Input: dimensioned drawing with shaded views. Units: mm. Origin: part minimum x, y, z. A direction names the side the tool comes from. Give positions to 0.01 mm unless a question says otherwise; leave off trailing zeros. Write each loop counter-clockwise with the first axis right and the second up, starting at its lowest first coordinate (ties: lowest second). Pieces come first, ordered by that corner, then holes. Notation, with made-up numbers: M -32.75,-15.75 L -12.75,-15.75 A23 ccw -12.75,16.25 Z; hole C -6,55.5 d7. An arc over 180 degrees is marked long. Use CSV: the item, a comma, the result in double quotes. Start each with the question number.
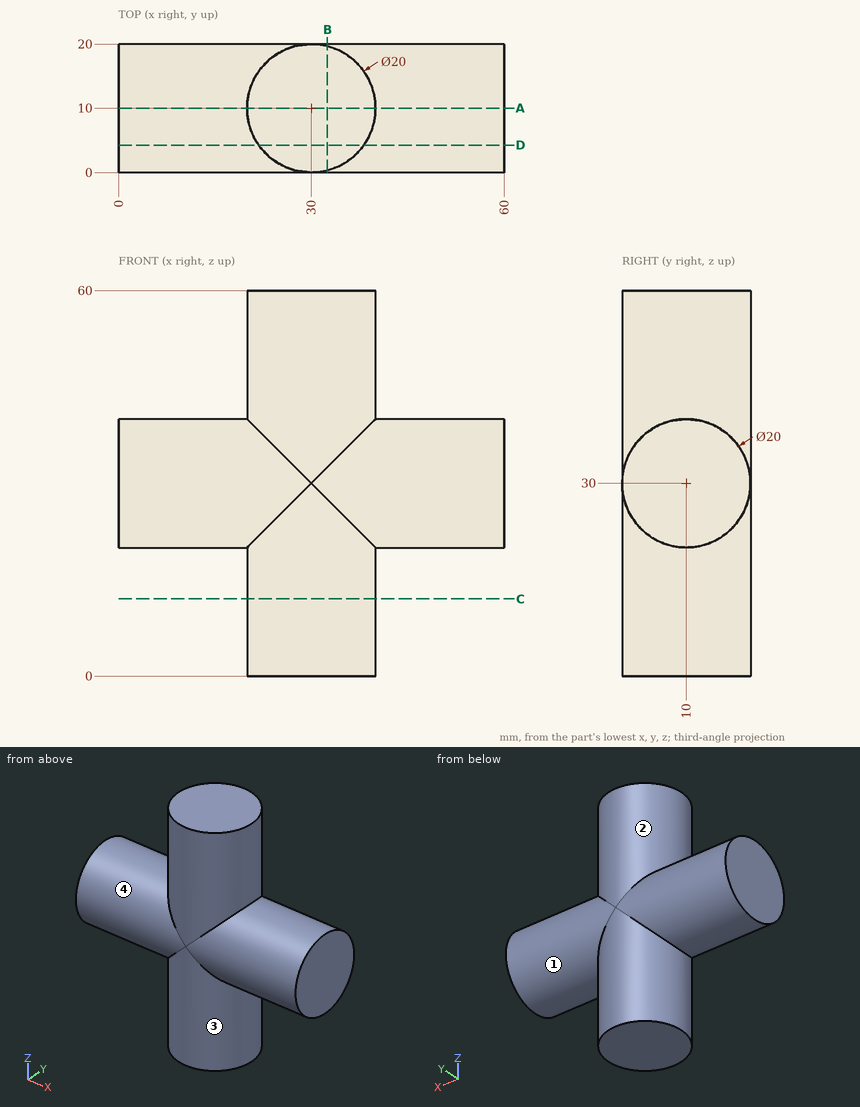
Q1. Set-up query: the marked faces 1, 2, 3 and 4. Return all of +Z, -Z, +X, -X, +Y, -Y with unobstructed straight access to the full face (end or side cutting, diameter ignored); none if empty.
Q2. Section C-C, the plane z = 12. Return the cut outline in (x, y).
Q3. Section A-A, the plane y = 10. Return the cut outline in (x, z), and give its area (3 significant figures).
Q4. Section D-D, the plane y = 4.25. Return the cut outline in (x, z).
Q5. First-contact query: pin 1 Ø12 at (y, z) = (5, 6.5) entering from +X; pin 2 Ø1.5 at (y, z) = (13, 37.5) entering from -X; pin 3 Ø3 at (y, z) = (13, 51.5) entering from +X; pin 4 Ø2 at (x, y) = (47, 10) entering from -Z. Flat tips, straight axial feed; report the tip coordinate or a pass-through.
Q6. Section B-B, the plane x = 32.5. Return the cut outline in (y, z).
Q7. Material intervals for L1, parallel to Y at x = 30.5, z = 46; L2, parallel to X at y = 14, z = 42.5; L3, parallel to X at y = 2.5, z = 50.5, sorted ascending. Write a range as [from, to].
Check result:
1,face 1,"+X"
1,face 2,"+Z"
1,face 3,"-Z"
1,face 4,"-X"
2,outline,"C 30,10 d20"
3,outline,"M 0,20 L 20,20 L 20,0 L 40,0 L 40,20 L 60,20 L 60,40 L 40,40 L 40,60 L 20,60 L 20,40 L 0,40 Z"
3,area,"2,000 mm²"
4,outline,"M 0,21.82 L 21.82,21.82 L 21.82,0 L 38.18,0 L 38.18,21.82 L 60,21.82 L 60,38.18 L 38.18,38.18 L 38.18,60 L 21.82,60 L 21.82,38.18 L 0,38.18 Z"
5,pin 1,"stops at x = 40"
5,pin 2,"stops at x = 0"
5,pin 3,"stops at x = 39.89"
5,pin 4,"stops at z = 20"
6,outline,"M 0.32,0 L 19.68,0 L 19.68,27.5 A10 ccw 19.68,32.5 L 19.68,60 L 0.32,60 L 0.32,32.5 A10 ccw 0.32,27.5 Z"
7,L1,"y = [0.01, 19.99]"
7,L2,"x = [20.83, 39.17]"
7,L3,"x = [23.39, 36.61]"
